Design review of the part built by this model. Coordinates are the model's own, in mm. Face numbers are marked on the shaded views. A direction names the side the tool comes from. Give positions to 0.01 mm unless a question says otherwise; leave off trailing zeros. Loops run counter-clockwise (first coordinate to the right, second up) from the corner with the lowest first, then second, coordinate; pieces in that order, holes last. Notation, with made-up numbers: (64.5, -19.5) -> (108.5, -19.5) arc R23 ccw to (108.5, -9.5) -> close; hole circle Ø1 at (-11.5, 74.5). An arc over 180 degrees is marked (long way). Use CSV: the item, a comma, the result in double quotes. Start each with the question number.
Item 1: Wall thickness on line 1 along Z through (x, y) = (10, -1.75); line 2 along X through (y, z) = (4.5, -69.5); line 3 along X through (y, z) = (6.5, 162.5): over which ranges is each line inside the solid? List them lowest first. Write a range as from..to.
Item 2: Clearance check with flat-ended pins moving along their axes: pin 1 (0.9 mm diameter, centred on x = -2, y = 10.5, fed in from -Z); pin 2 (1.5 mm diameter, centred on x = -2, z = -9.5, fed in from +Y); pin 3 (2 mm diameter, centred on y = -3, z = -45, fed in from +X); pin 4 (12 mm diameter, centred on y = 6, z = -54.5, fed in from -X). State where each tip first meets the part, or that it passes through.
Item 3: We need section B-B (x = 0). State the section outline as (y, z) points, plus the area to 3 significant figures.
Item 4: For the marked faces 1, 2 and 3, list the 3-axis set-ups (+Z, -Z, +X, -X, +Y, -Y) from which the entire face can be reached by the end or side of a thin tool; tool diameter is ignored.
Item 5: We need section C-C (z = 127.5). State the section outline as (x, y) points.
Item 6: We need section D-D (z = -32). State the section outline as (x, y) points, plus the area to 3 significant figures.
Item 7: We need section A-A (y = 0). State the section outline as (x, z) points.
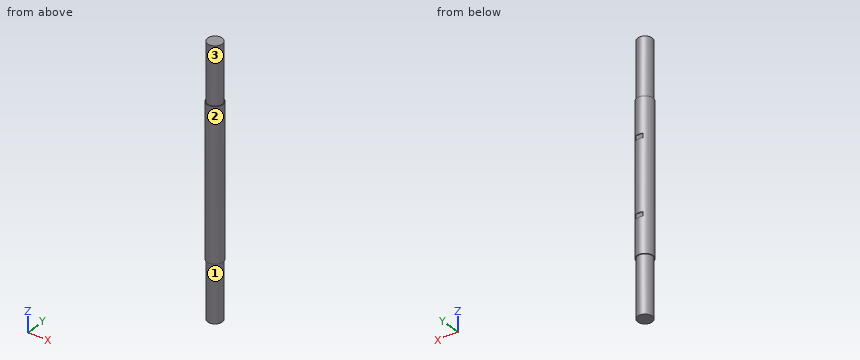
from build123d import *

# Parameters (mm, degrees)
SKETCH1_W          = 360
SKETCH1_H          = 11
SKETCH4_W          = 6
SKETCH4_H          = 10
CUT_EXTRUDE1_DEPTH = 181.670971658
SKETCH6_W          = 78
SKETCH6_H          = 1


with BuildPart() as part:
    # Sketch1 → Revolve1 (revolve)
    with BuildSketch(Plane(origin=(0, 0, 0), x_dir=(0, 0, -1), z_dir=(1, 0, 0)), mode=Mode.PRIVATE) as revolve1_sk:
        with Locations((0, 5.5)):
            Rectangle(SKETCH1_W, SKETCH1_H)
    revolve(revolve1_sk.sketch.rotate(Axis((0, 0, -180), (0, 0, 1)), 90), axis=Axis((0, 0, -180), (0, 0, 1)))

    # Sketch4 → Cut-Extrude1 (cut, symmetric)
    with BuildSketch(Plane(origin=(0, 0, 0), x_dir=(0, 0, -1), z_dir=(1, 0, 0))):
        with Locations((-50.8, 14.92)):
            Rectangle(SKETCH4_W, SKETCH4_H)
    cut_extrude1 = extrude(amount=CUT_EXTRUDE1_DEPTH, both=True, mode=Mode.SUBTRACT)

    # Sketch6 → Cut-Revolve1 (revolve, cut)
    with BuildSketch(Plane(origin=(0, 0, 0), x_dir=(0, 0, -1), z_dir=(1, 0, 0)), mode=Mode.PRIVATE) as cut_revolve1_sk:
        with Locations((-141, 10.5)):
            Rectangle(SKETCH6_W, SKETCH6_H)
    cut_revolve1 = revolve(cut_revolve1_sk.sketch.rotate(Axis((0, 0, -180), (0, 0, -1)), 270), axis=Axis((0, 0, -180), (0, 0, -1)), mode=Mode.SUBTRACT)

    # Mirror2: Cut-Extrude1, Cut-Revolve1 across plane
    add(cut_extrude1.mirror(Plane.XY), mode=Mode.SUBTRACT)
    add(cut_revolve1.mirror(Plane.XY), mode=Mode.SUBTRACT)


solid = part.part
Results found:
1,line 1,"-102..102"
1,line 2,"-10.04..10.04"
1,line 3,"-7.6..7.6"
2,pin 1,"z = -102"
2,pin 2,"y = 10.93"
2,pin 3,"x = 10.82"
2,pin 4,"x = -11"
3,outline,"(-11, -102) -> (-10, -102) -> (-10, -180) -> (10, -180) -> (10, -102) -> (11, -102) -> (11, -53.8) -> (9.92, -53.8) -> (9.92, -47.8) -> (11, -47.8) -> (11, 47.8) -> (9.92, 47.8) -> (9.92, 53.8) -> (11, 53.8) -> (11, 102) -> (10, 102) -> (10, 180) -> (-10, 180) -> (-10, 102) -> (-11, 102) -> close"
3,area,"7,600 mm²"
4,face 1,"-Z"
4,face 2,"+Z, -Z"
4,face 3,"+Z"
5,outline,"circle Ø20 at (0, 0)"
6,outline,"circle Ø22 at (0, 0)"
6,area,"380 mm²"
7,outline,"(-11, -102) -> (-10, -102) -> (-10, -180) -> (10, -180) -> (10, -102) -> (11, -102) -> (11, 102) -> (10, 102) -> (10, 180) -> (-10, 180) -> (-10, 102) -> (-11, 102) -> close"
